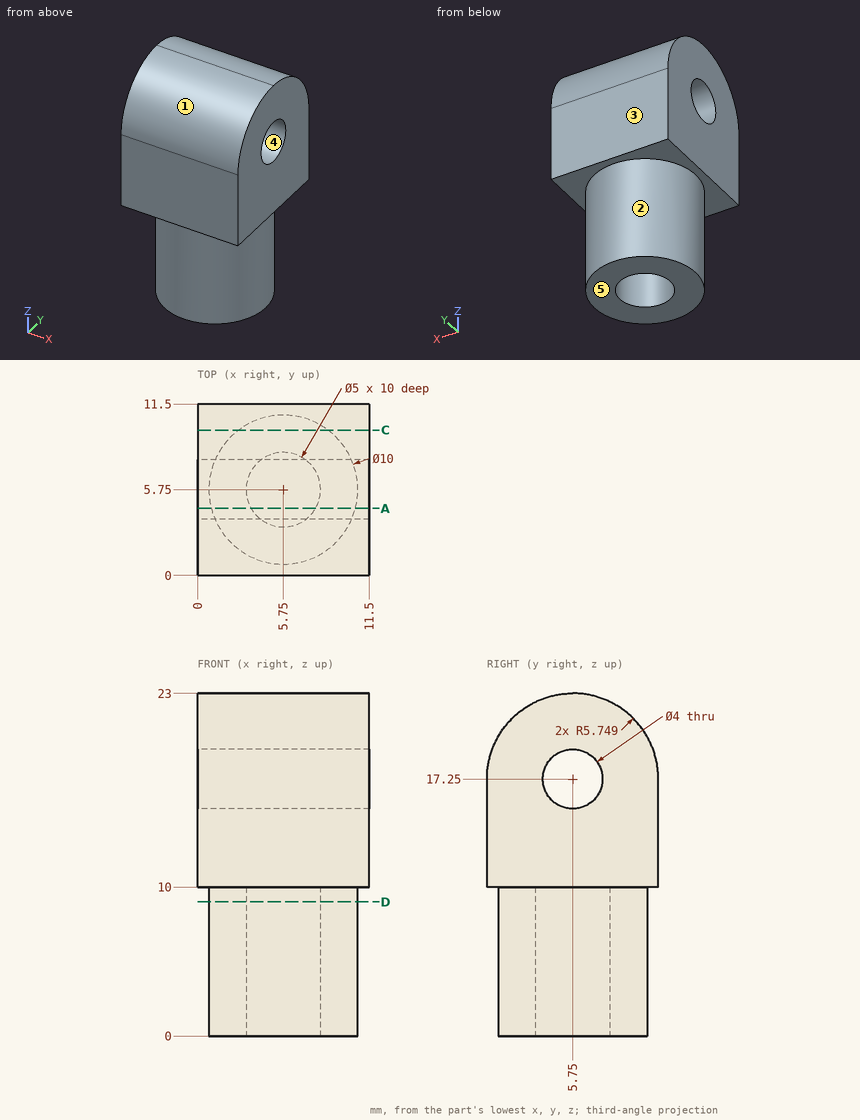
Verification items for this drawing (mm, ordinates from the low corner). A direction names the side the tool comes from. Round coordinates to 2 decimals unless told otherwise and drop trailing zeros. Order: outer loops, then holes, each group sorted by start corner. A loop starts at its lowest first (then second) coordinate and runs counter-clockwise, first axis right, second up. Notation, with made-up numbers: (74.25, 53.25) -> (126.25, 53.25) arc R18 cw to (126.25, 57.25) -> close; hole circle Ø2 at (-10.75, -33.5). An arc over 180 degrees is marked (long way). Use one line per item in the form item = value.
1. Cross-section at D-D, the plane z = 9. Enter the section's corners in (x, y).
Working result:
outline = circle Ø10 at (5.75, 5.75); hole circle Ø5 at (5.75, 5.75)
2. Set-up check for the marked faces 1 and 2: record each of +Z, -Z, +X, -X, +Y, -Y from which the full face is reachable in a straight line by a thin tool's end or side.
Working result:
face_1 = +Z, +X, -X, -Y
face_2 = -Z
3. Cross-section at C-C, the plane y = 9.75. Enter the section's corners in (x, z), plus the area to 3 significant figures.
Working result:
outline = (0, 10) -> (2.75, 10) -> (2.75, 0) -> (8.75, 0) -> (8.75, 10) -> (11.5, 10) -> (11.5, 21.38) -> (0, 21.38) -> close
area = 191 mm^2
4. Scan lines: line 1 along Z through (x, y) = (8.75, 5.75); line 2 along Z through (x, y) = (6.25, 5.75); line 3 along Y through (x, z) = (5, 17.25). Record each from-to range of solid material in increasing order. Write a range as from..to.
Working result:
line_1 = 0..15.25, 19.25..23
line_2 = 10..15.25, 19.25..23
line_3 = 0..3.75, 7.75..11.5
5. Cross-section at A-A, the plane y = 4.5. Enter the section's corners in (x, z) (1 decimal), plus the area to 3 significant figures.
Working result:
outline = (0, 10) -> (0.9, 10) -> (0.9, 0) -> (3.6, 0) -> (3.6, 10) -> (7.9, 10) -> (7.9, 0) -> (10.6, 0) -> (10.6, 10) -> (11.5, 10) -> (11.5, 15.7) -> (0, 15.7) -> close; (0, 18.8) -> (11.5, 18.8) -> (11.5, 22.9) -> (0, 22.9) -> close
area = 166 mm^2
6. Go/stop test with flat-tipped pins: pin 1 (4 mm diameter, centred on x = 6.5, y = 5.5, fed in from -Z); pin 2 (1.5 mm diameter, centred on x = 2.5, z = 6.5, fed in from -Y); pin 3 (5 mm diameter, centred on y = 9, z = 3.5, fed in from -X); pin 4 (2 mm diameter, centred on x = 9, z = 8.5, fed in from +Y) (1 decimal). Record where each tip stops, or that it passes through.
Working result:
pin_1 = 0
pin_2 = 1.42
pin_3 = 0.81
pin_4 = 10.2
7. Mould release check, pull along Z, two halves, no side actions. Record for the marked faces 3, 4 and 5: pulls with the +Z half, pulls with the -Z half, needs draft (parallel to the pull), parting line crosses it, or undercut.
Working result:
face_3 = needs draft
face_4 = undercut
face_5 = pulls with the -Z half
